Autodesk Inventor part; units mm, degrees
ref_plane "YZ Plane" through (0, 0, 0) normal (1, 0, 0) x (0, 1, 0)
ref_plane "XZ Plane" through (0, 0, 0) normal (0, 1, 0) x (-1, 0, 0)
ref_plane "XY Plane" through (0, 0, 0) normal (0, 0, 1) x (1, 0, 0)
sketch "Sketch1" plane through (0, 0, 0) normal (0, 1, 0) x (-1, 0, 0)
  line L0 (0, 0) -> (200, 0)
  line L1 (200, 0) -> (200, -200)
  line L2 (200, -200) -> (0, -200)
  line L3 (0, -200) -> (0, 0)
  dimension "d0" = 200
  dimension "d1" = 200
extrude "Extrusion1" add sketch "Sketch1" along normal blind 2
fillet "Fillet1" radius 20 4 edges at (-200, 1, 0) (0, 1, 0) (0, 1, -200) (-200, 1, -200)
sketch "Sketch4" plane through (0, 2, 0) normal (0, 1, 0) x (1, 0, 0)
  arc A0 (-20, 0) -> (0, 20) centre (-20, 20) ccw
  arc A1 (-200, 20) -> (-180, 0) centre (-180, 20) ccw
  arc A2 (0, 180) -> (-20, 200) centre (-20, 180) ccw
  arc A3 (-180, 200) -> (-200, 180) centre (-180, 180) ccw
  circle A4 centre (-20, 180) radius 2.5
  circle A5 centre (-180, 180) radius 2.5
  circle A6 centre (-180, 20) radius 2.5
  circle A7 centre (-20, 20) radius 2.5
  line L0 (-180, 0) -> (-20, 0)
  line L1 (0, 20) -> (0, 180)
  point P0 (0, 0)
  dimension "d19" = 5
  dimension "d20" = 5
  dimension "d21" = 5
  dimension "d22" = 5
extrude "Extrusion4" cut sketch "Sketch4" against normal blind 2
sketch "Sketch6" plane through (0, 2, 0) normal (0, 1, 0) x (1, 0, 0)
  circle A0 centre (-100, 70) radius 2.5
  circle A1 centre (-100, 130) radius 2.5
  point P0 (0, 0)
  dimension "d34" = 5
  dimension "d35" = 5
extrude "Extrusion6" cut sketch "Sketch6" against normal blind 10
properties part number "Basequadrada" material "PPS Plastic"
The model under review builds one solid part; all positions refer to its coordinate system, in mm. Round coordinates to 2 decimals unless told otherwise and drop trailing zeros. Loops run counter-clockwise (first coordinate to the right, second up) from the corner with the lowest first, then second, coordinate; pieces in that order, holes last. Notation, with made-up numbers: (-23, -27) - (33, -27) arc R3 cw to (33, -23) - close; hole circle Ø11 at (56.25, 71). An arc over 180 degrees is marked (long way). Use a Markdown table: item, result. Add a question column.
Q1. Add section A-A (z = -130). State the section outline as (x, y) points.
Q2. Insertion check: pin 1 Ø4.5 at (x, z) = (-20, -180) entering from +Y. The pin has a flat end and moves straight along its axis. Give the tip position at first contact, or say it passes through.
Q3. For probe 1 along X at (y, z) = (1.25, -180); probe 2 along Z at (x, y) = (-100, 0.55), list the stretches that pass through material, from the lowest coordinate up.
Q4. The part is to be moulded in two halves that separate along X. For faces 1 (the face through (-178.66, 1.01, -182.11)), 2 (the face through (-193.986, 1.014, -194.297)), 3 (the face through (-99, 2, -99)), say which applies: pulls with the +X half, pulls with the -X half, needs draft (parallel to the pull), parting line crosses it, or undercut.
Worked answers:
| question | item | result |
|---|---|---|
| 1 | outline | (-200, 0) - (-102.5, 0) - (-102.5, 2) - (-200, 2) - close; (-97.5, 0) - (0, 0) - (0, 2) - (-97.5, 2) - close |
| 2 | pin 1 | through |
| 3 | probe 1 | -200 to -182.5, -177.5 to -22.5, -17.5 to 0 |
| 3 | probe 2 | -200 to -132.5, -127.5 to -72.5, -67.5 to 0 |
| 4 | face 1 | undercut |
| 4 | face 2 | pulls with the -X half |
| 4 | face 3 | needs draft |
